Check sheet for the modelled part. Datum: model origin and axes. Units: mm. Coordinates: 2 decimals unless noted, no trailing zeros. Loops run counter-clockwise (first coordinate to the right, second up) from the corner with the lowest first, then second, coordinate; pieces in that order, holes last. Notation, with made-up numbers: (8.25, 73.5) - (32.25, 73.5) arc R17 ccw to (32.25, 85.5) - close; hole circle Ø2 at (46.25, 8.5). An arc over 180 degrees is marked (long way). Write each question's results on one line, items separated by ' | '. Start each with the question number.
1. Cross-section at B-B (x = 0). Record the cut outline in (y, z), and give its area (3 significant figures).
2. Cross-section at C-C (x = 26). Record the cut outline in (y, z), and give its area (3 significant figures).
3. Thickness scan on line 1 (Y direction, x = 21, z = 1); line 2 (X direction, y = 16, z = 2.2); line 3 (Y direction, x = -22.5, z = 2.15). Record the ranges inside material, lowest first. Write a range as [from, to].
4. Cross-section at D-D (y = 30.5). Record the cut outline in (x, z), and give its area (3 significant figures).
5. Cross-section at A-A (y = -17.5). Record the cut outline in (x, z), and give its area (3 significant figures).
6. Gauge pin test, flat end, axial feed: P1, Ø1.5, axis at x = 43, z = 1, coming from the +Y side. Record the tip position at first contact, or that the pin passes through.
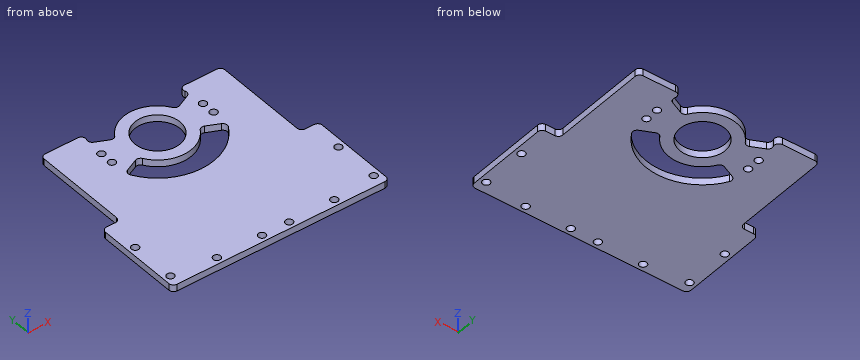
```python
from build123d import *

# Parameters (mm, degrees)
SKETCH_1_W          = 80
SKETCH_1_H          = 85
SKETCH_1_R          = 10
SKETCH_1_R_2        = 1.65
EXTRUDE_1_DEPTH     = 3
CUT_EXTRUDE_1_DEPTH = 59.440140315
SKETCH_3_W          = 8
SKETCH_3_H          = 40
EXTRUDE_2_DEPTH     = 3
SKETCH_4_R          = 1.65
CUT_EXTRUDE_2_DEPTH = 65.181383594
FILLET_1_R          = 2
FILLET_2_R          = 2


with BuildPart() as part:
    # 草图1 → 凸台-拉伸1 (new body)
    with BuildSketch(Plane.XY):
        Rectangle(SKETCH_1_W, SKETCH_1_H)
        with Locations((0, 27.5)):
            Circle(SKETCH_1_R, mode=Mode.SUBTRACT)
        with Locations((-6, -39.5)):
            Circle(SKETCH_1_R_2, mode=Mode.SUBTRACT)
        with Locations((-26, -39.5)):
            Circle(SKETCH_1_R_2, mode=Mode.SUBTRACT)
        with Locations(Location((26, -39.5, 0), (0, 0, 180))):
            Circle(SKETCH_1_R_2, mode=Mode.SUBTRACT)
        with Locations(Location((6, -39.5, 0), (0, 0, 180))):
            Circle(SKETCH_1_R_2, mode=Mode.SUBTRACT)
        with Locations((-22.5, 30.5)):
            Circle(SKETCH_1_R_2, mode=Mode.SUBTRACT)
        with Locations(Location((-22.5, 24.5, 0), (0, 0, 180))):
            Circle(SKETCH_1_R_2, mode=Mode.SUBTRACT)
        with Locations(Location((22.5, 30.5, 0), (0, 0, 180))):
            Circle(SKETCH_1_R_2, mode=Mode.SUBTRACT)
        with Locations((22.5, 24.5)):
            Circle(SKETCH_1_R_2, mode=Mode.SUBTRACT)
    extrude(amount=EXTRUDE_1_DEPTH)

    # 草图2 → 切除-拉伸1 (cut, through all)
    with BuildSketch(Plane.XY.offset(3)):
        with BuildLine():
            Line((22.657694676, 16.934543456), (13.594616806, 21.160726074))
            ThreePointArc((13.594616806, 21.160726074), (0, 12.5), (-13.594616806, 21.160726074))
            Line((-13.594616806, 21.160726074), (-22.657694676, 16.934543456))
            ThreePointArc((-22.657694676, 16.934543456), (0, 2.5), (22.657694676, 16.934543456))
        make_face()
        with BuildLine():
            Line((-22.657694676, 38.065456544), (-13.594616806, 33.839273926))
            ThreePointArc((-13.594616806, 33.839273926), (0, 42.5), (13.594616806, 33.839273926))
            Line((13.594616806, 33.839273926), (22.657694676, 38.065456544))
            ThreePointArc((22.657694676, 38.065456544), (0, 52.5), (-22.657694676, 38.065456544))
        make_face()
    extrude(amount=-CUT_EXTRUDE_1_DEPTH, mode=Mode.SUBTRACT)

    # 草图3 → 凸台-拉伸2 (add)
    with BuildSketch(Plane.XY.offset(3)):
        with Locations((44, -22.5)):
            Rectangle(SKETCH_3_W, SKETCH_3_H)
        with Locations((-44, -22.5)):
            Rectangle(SKETCH_3_W, SKETCH_3_H)
    extrude(amount=-EXTRUDE_2_DEPTH)

    # 草图4 → 切除-拉伸2 (cut, through all)
    with BuildSketch(Plane.XY.offset(3)):
        with Locations((45, -37.5)):
            Circle(SKETCH_4_R)
        with Locations((45, -17.5)):
            Circle(SKETCH_4_R)
        with Locations(Location((-45, -17.5, 0), (0, 0, 180))):
            Circle(SKETCH_4_R)
        with Locations(Location((-45, -37.5, 0), (0, 0, 180))):
            Circle(SKETCH_4_R)
    extrude(amount=-CUT_EXTRUDE_2_DEPTH, mode=Mode.SUBTRACT)

    # 圆角1
    fillet_1_edges = [part.edges().sort_by_distance(p)[0] for p in [
        (-48, -2.5, 1.5),
        (-13.594616806, 21.160726074, 1.5),
        (13.594616806, 21.160726074, 1.5),
        (22.657694676, 16.934543456, 1.5),
        (-22.657694676, 16.934543456, 1.5),
        (-22.657694676, 38.065456544, 1.5),
        (13.594616806, 33.839273926, 1.5),
        (22.657694676, 38.065456544, 1.5),
        (-13.594616806, 33.839273926, 1.5),
        (-40, 42.5, 1.5),
        (40, -2.5, 1.5),
        (48, -2.5, 1.5),
    ]]
    fillet(fillet_1_edges, radius=FILLET_1_R)

    # 圆角2
    fillet_2_edges = [part.edges().sort_by_distance(p)[0] for p in [
        (20, 42.5, 1.5),
        (-20, 42.5, 1.5),
        (40, 42.5, 1.5),
        (-48, -42.5, 1.5),
        (48, -42.5, 1.5),
        (-40, -2.5, 1.5),
    ]]
    fillet(fillet_2_edges, radius=FILLET_2_R)


solid = part.part
```
Established:
1) outline: (-42.5, 0) - (2.5, 0) - (2.5, 3) - (-42.5, 3) - close; (12.5, 0) - (17.5, 0) - (17.5, 3) - (12.5, 3) - close; (37.5, 0) - (42.5, 0) - (42.5, 3) - (37.5, 3) - close | area: 165 mm^2
2) outline: (-42.5, 0) - (-41.15, 0) - (-41.15, 3) - (-42.5, 3) - close; (-37.85, 0) - (42.5, 0) - (42.5, 3) - (-37.85, 3) - close | area: 245 mm^2
3) line 1: [-42.5, 13.94], [17.69, 23.81], [25.19, 29.81], [31.19, 37.31] | line 2: [-40, -21.92], [-9.63, 9.63], [21.92, 40] | line 3: [-42.5, 22.85], [26.15, 28.85], [32.15, 42.15]
4) outline: (-40, 0) - (-24.15, 0) - (-24.15, 3) - (-40, 3) - close; (-20.85, 0) - (-9.54, 0) - (-9.54, 3) - (-20.85, 3) - close; (9.54, 0) - (20.85, 0) - (20.85, 3) - (9.54, 3) - close; (24.15, 0) - (40, 0) - (40, 3) - (24.15, 3) - close | area: 163 mm^2
5) outline: (-48, 0) - (-46.65, 0) - (-46.65, 3) - (-48, 3) - close; (-43.35, 0) - (43.35, 0) - (43.35, 3) - (-43.35, 3) - close; (46.65, 0) - (48, 0) - (48, 3) - (46.65, 3) - close | area: 268 mm^2
6) P1: y = -2.5
